Part model, mm, in its own coordinate system. Face numbers are marked on the shaded views. A direction names the side the tool comes from. Give positions to 0.01 mm unless a question says otherwise; leave off trailing zeros. Loops run counter-clockwise (first coordinate to the right, second up) from the corner with the lowest first, then second, coordinate; pieces in that order, holes last. Notation, with made-up numbers: (-32, -24.75) -> (24, -24.75) arc R30 ccw to (24, 2.25) -> close; hole circle Ø7 at (-35, 52). An arc over 180 degrees is marked (long way). One line per question, with ' | ' between items.
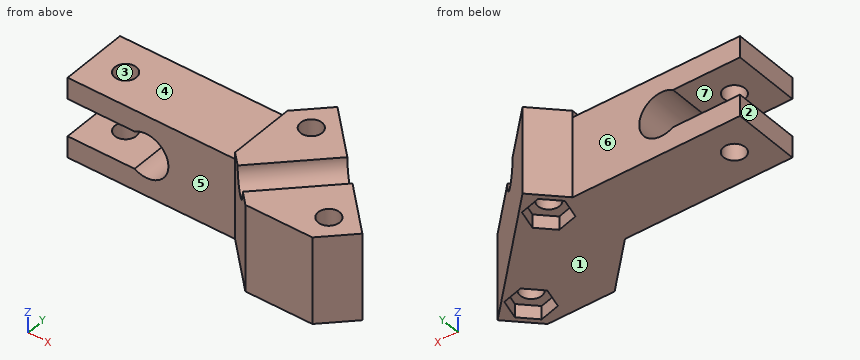
```python
from build123d import *

# Parameters (mm, degrees)
PAD_DEPTH            = 10
SKETCH_R             = 1.6
PAD001_DEPTH         = 7
PAD001_DEPTH_BACK    = 6
SKETCH004_R          = 2.5
POCKET_DEPTH         = 27.372693
POCKET001_DEPTH      = 2
SKETCH006_R          = 1.6
POCKET002_DEPTH      = 6.001
POCKET002_DEPTH_BACK = -7.001


with BuildPart() as part:
    # Sketch003 → Pad (new body)
    with BuildSketch(Plane.XZ):
        with BuildLine():
            Line((13.253575, -6), (-11.746425, -6))
            Line((-11.746425, -2.8), (-11.746425, -6))
            Line((-1.746425, -2.8), (-11.746425, -2.8))
            ThreePointArc((-1.746425, -2.8), (3.3, 0), (-1.746425, 2.8))
            Line((-1.746425, 2.8), (-11.746425, 2.8))
            Line((-11.746425, 2.8), (-11.746425, 6))
            Line((13.253575, 6), (-11.746425, 6))
            Line((13.253575, 6), (13.253575, 0))
            Line((13.253575, 0), (13.253575, -6))
        make_face()
    extrude(amount=PAD_DEPTH)

    # Sketch → Pad001 (join, two sides)
    with BuildSketch(Plane.XY) as pad001_sk:
        Polygon((13.253575, -10), (20.324643, -17.071068), (30.324643, -17.071068), (34.517031, -12.87868), (17.445963, 4.192388), (13.253575, 0), align=None)
        with Locations((17.445963, -0.807612)):
            Circle(SKETCH_R, mode=Mode.SUBTRACT)
        with Locations((29.517031, -12.87868)):
            Circle(SKETCH_R, mode=Mode.SUBTRACT)
    extrude(amount=PAD001_DEPTH)
    extrude(pad001_sk.sketch, amount=-PAD001_DEPTH_BACK)

    # Sketch004 (on DatumPlane) → Pocket (cut, through all)
    with BuildSketch(Plane(origin=(0, 0, 3.5), x_dir=(0, 0, -1), z_dir=(-0.707107, -0.707107, 0))):
        with Locations((-3.5, 21.442761)):
            Circle(SKETCH004_R)
    extrude(amount=-POCKET_DEPTH, mode=Mode.SUBTRACT)

    # Sketch005 (on DatumPlane) → Pocket001 (cut)
    with BuildSketch(Plane.XY.offset(-6)):
        Polygon((18.267824, -3.874838), (20.51319, -1.629473), (19.691329, 1.437754), (16.624102, 2.259615), (14.378737, 0.014249), (15.200598, -3.052977), align=None)
        Polygon((30.338892, -15.945906), (32.584257, -13.700541), (31.762397, -10.633314), (28.69517, -9.811453), (26.449805, -12.056819), (27.271665, -15.124045), align=None)
    extrude(amount=POCKET001_DEPTH, mode=Mode.SUBTRACT)

    # Sketch006 → Pocket002 (cut, two sides)
    with BuildSketch(Plane.XY) as pocket002_sk:
        with Locations((-7, -5)):
            Circle(SKETCH006_R)
    extrude(amount=-POCKET002_DEPTH, mode=Mode.SUBTRACT)
    extrude(pocket002_sk.sketch, amount=-POCKET002_DEPTH_BACK, mode=Mode.SUBTRACT)


solid = part.part
```
1) Pin check, flat tips, straight feed: P1, Ø2, axis at y = -8.5, z = -2, coming from the +X side; P2, Ø3, axis at x = 14, z = 3.5, coming from the -Y side; P3, Ø4, axis at x = 17.45, y = -0.81, coming from the -Z side. Stop position of each tip, or through.
Found:
P1: x = 31.14 | P2: y = -12.25 | P3: z = -4
2) Saw through at A-A (x = 0). Give the cut face in (y, z), and give its area (3 significant figures).
Found:
outline: (-10, -6) -> (0, -6) -> (0, -3.3) -> (-10, -3.3) -> close; (-10, 3.3) -> (0, 3.3) -> (0, 6) -> (-10, 6) -> close | area: 54.0 mm2
3) Pull direction X, two halves, no side cores. Call the marked faces 1, 2 and 3: pulls with the +X half, pulls with the -X half, needs draft (parallel to the pull), parting line crosses it, or undercut.
Found:
face 1: needs draft | face 2: pulls with the -X half | face 3: undercut
4) Saw through at D-D (y = -5). State how many separate pieces and enclosed holes the cut face has, and give its area (3 significant figures).
Found:
separate pieces: 3 | enclosed holes: 0 | area: 359 mm2
5) Saw through at C-C (z = 0). Give the cut face in (x, y).
Found:
outline: (3.3, -10) -> (13.25, -10) -> (20.32, -17.07) -> (30.32, -17.07) -> (34.52, -12.88) -> (17.45, 4.19) -> (13.25, 0) -> (3.3, 0) -> close; hole circle Ø3.2 at (17.45, -0.81); hole circle Ø3.2 at (29.52, -12.88)
6) Drill centre lines: line 1 (Z direction, x = -7, y = -1); line 2 (Y direction, x = -7, z = 4.8); line 3 (Y direction, x = 9, z = -2). Where is each one in solid material? Low to high.
Found:
line 1: -6 to -2.8, 2.8 to 6 | line 2: -10 to -6.6, -3.4 to 0 | line 3: -10 to 0
7) Saw through at B-B (x = -7). Give the cut face in (y, z), and give its area (3 significant figures).
Found:
outline: (-10, -6) -> (-6.6, -6) -> (-6.6, -2.8) -> (-10, -2.8) -> close; (-10, 2.8) -> (-6.6, 2.8) -> (-6.6, 6) -> (-10, 6) -> close; (-3.4, -6) -> (0, -6) -> (0, -2.8) -> (-3.4, -2.8) -> close; (-3.4, 2.8) -> (0, 2.8) -> (0, 6) -> (-3.4, 6) -> close | area: 43.5 mm2
8) Tool access for the marked faces 4, 5, 6 and 7: list every direction of +Z, -Z, +X, -X, +Y, -Y with a clear straight run to the whole face (end or side of a thin tool).
Found:
face 4: +Z, -X, +Y, -Y | face 5: +Z, -Z, -X, -Y | face 6: +Z, -Z, -X, +Y | face 7: -X, +Y, -Y
